Verification items for the finished model (mm, model axes). Face numbers are marked on the shaded views. Give positions to 0.01 mm unless a question says otherwise; leave off trailing zeros. Loops run counter-clockwise (first coordinate to the right, second up) from the corner with the lowest first, then second, coordinate; pieces in that order, holes last. Notation, with made-up numbers: (-38.5, -9) - (-21.5, -9) arc R35 cw to (-21.5, 25) - close; hole circle Ø3 at (5, 59). An arc over 180 degrees is marked (long way). One line per question, with ' | ' between items. Start each with the question number.
1. Depth check by flat-ended pin: pin 1 Ø1.5 at (y, z) = (15, 1) entering from -X; pin 2 Ø1.1 at (x, z) = (20.5, 1.5) entering from +Y; pin 3 Ø0.7 at (x, z) = (-20, 1.5) entering from -Y. Enter the tip coordinate at first touch or a pass-through.
2. Section check B-B, the plane z = 0.6. Enter the section's corners in (x, y), then the cut area to 3 significant figures.
3. Thickness scan on line 1 along Y through (x, z) = (0, 0.9); line 2 along Y through (x, z) = (17.5, 1.2); line 3 along Y through (x, z) = (16.5, 0.5). Record the ranges inside material, lowest first. Write a range as from..to.
4. Section check A-A, the plane y = 7. Enter the section's corners in (x, z), then the cut area to 3 significant figures.
5. Section check D-D, the plane y = 19.5. Enter the section's corners in (x, z).
6. Section check C-C, the plane y = 14.5. Enter the section's corners in (x, z).
7. Mould release check, pull along X, two halves, no side actions. Record for the marked faces 1, 2 and 3: +X half, -X half, draft (parallel to the pull), parting line (faces both ways), or undercut.
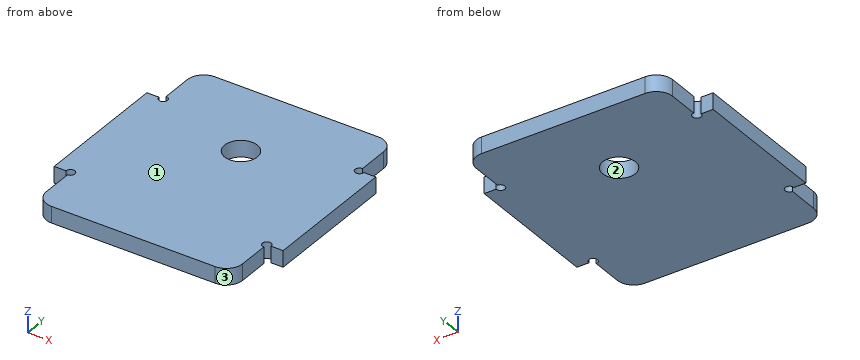
from build123d import *

# Parameters (mm, degrees)
SKETCH1_W           = 3
SKETCH1_H           = 25
BOSS_EXTRUDE1_DEPTH = 3
SKETCH5_R           = 3
CUT_EXTRUDE3_DEPTH  = 31.56141358
SKETCH6_R           = 0.8
CUT_EXTRUDE4_DEPTH  = 31.56141358
FILLET1_R           = 3


with BuildPart() as part:
    # Sketch1 → Boss-Extrude1 (new body)
    with BuildSketch(Plane.XY):
        Polygon((-18, -12.5), (-18, -22), (18, -22), (18, -12.5), (15, -12.5), (15, 12.5), (18, 12.5), (18, 22), (-18, 22), (-18, 12.5), (-15, 12.5), (-15, -12.5), align=None)
        with Locations((-19.5, 0)):
            Rectangle(SKETCH1_W, SKETCH1_H)
        with Locations((-16.5, 0)):
            Rectangle(SKETCH1_W, SKETCH1_H)
        with Locations((19.5, 0)):
            Rectangle(SKETCH1_W, SKETCH1_H)
        with Locations((16.5, 0)):
            Rectangle(SKETCH1_W, SKETCH1_H)
    extrude(amount=BOSS_EXTRUDE1_DEPTH)

    # Sketch5 → Cut-Extrude3 (cut, through all)
    with BuildSketch(Plane(origin=(0, 0, 0), x_dir=(-1, 0, 0), z_dir=(0, 0, -1))):
        with Locations((0, 7)):
            Circle(SKETCH5_R)
    extrude(amount=-CUT_EXTRUDE3_DEPTH, mode=Mode.SUBTRACT)

    # Sketch6 → Cut-Extrude4 (cut, through all)
    with BuildSketch(Plane(origin=(0, 0, 0), x_dir=(-1, 0, 0), z_dir=(0, 0, -1))):
        with Locations((-18, 12.5)):
            Circle(SKETCH6_R)
        with Locations((-18, -12.5)):
            Circle(SKETCH6_R)
        with Locations((18, -12.5)):
            Circle(SKETCH6_R)
        with Locations((18, 12.5)):
            Circle(SKETCH6_R)
    extrude(amount=-CUT_EXTRUDE4_DEPTH, mode=Mode.SUBTRACT)

    # Fillet1
    fillet1_edges = [part.edges().sort_by_distance(p)[0] for p in [
        (-18, 22, 1.5),
        (18, 22, 1.5),
        (18, -22, 1.5),
        (-18, -22, 1.5),
    ]]
    fillet(fillet1_edges, radius=FILLET1_R)


solid = part.part
Results list:
1) pin 1: x = -18 | pin 2: y = 12.5 | pin 3: y = -12.5
2) outline: (-21, -12.5) - (-18.8, -12.5) arc R0.8 cw (long way) to (-18, -13.3) - (-18, -19) arc R3 ccw to (-15, -22) - (15, -22) arc R3 ccw to (18, -19) - (18, -13.3) arc R0.8 cw (long way) to (18.8, -12.5) - (21, -12.5) - (21, 12.5) - (18.8, 12.5) arc R0.8 cw (long way) to (18, 13.3) - (18, 19) arc R3 ccw to (15, 22) - (-15, 22) arc R3 ccw to (-18, 19) - (-18, 13.3) arc R0.8 cw (long way) to (-18.8, 12.5) - (-21, 12.5) - close; hole circle Ø6 at (0, 7) | area: 1,690 mm²
3) line 1: -22..4, 10..22 | line 2: -20.66..-13.12, -11.88..11.88, 13.12..20.66 | line 3: -21.6..21.6
4) outline: (-21, 0) - (-3, 0) - (-3, 3) - (-21, 3) - close; (3, 0) - (21, 0) - (21, 3) - (3, 3) - close | area: 108 mm²
5) outline: (-17.96, 0) - (17.96, 0) - (17.96, 3) - (-17.96, 3) - close
6) outline: (-18, 0) - (18, 0) - (18, 3) - (-18, 3) - close
7) face 1: draft | face 2: undercut | face 3: +X half
